Autodesk Inventor part; units mm, degrees
ref_plane "Work Plane1" through (0, 0, -15) normal (0, 0, 1) x (1, 0, 0)
ref_plane "YZ Plane" through (0, 0, 0) normal (1, 0, 0) x (0, 1, 0)
ref_plane "XZ Plane" through (0, 0, 0) normal (0, 1, 0) x (-1, 0, 0)
sketch "Sketch1" plane through (0, 0, 0) normal (0, 0, 1) x (1, 0, 0)
  line L0 (0, 0) -> (25, 0)
  line L1 (25, 0) -> (25, 40)
  line L2 (25, 40) -> (0, 40)
  line L3 (0, 40) -> (0, 0)
  dimension "d1" = 25
  dimension "d2" = 40
  dimension "d3" = 25
extrude "Extrusion1" add sketch "Sketch1" against normal blind 30
sketch "Sketch2" plane through (25, 0, 0) normal (1, 0, 0) x (0, 0, -1)
  line L0 (0, 0) -> (30, 0)
  circle A0 centre (15, 6.56) radius 2.46
extrude "Extrusion2" cut sketch "Sketch2" against normal blind 30
sketch "Sketch3" plane through (0, 0, 0) normal (-1, 0, 0) x (0, 0, 1)
  line L0 (0, 0) -> (-30, 0)
  line L1 (-25.05, 0) -> (-4.95, 0)
  line L2 (-4.95, 0) -> (-4.95, 33.12)
  line L3 (-4.95, 33.12) -> (-25.05, 33.12)
  line L4 (-25.05, 33.12) -> (-25.05, 0)
  dimension "d11" = 20.1
extrude "Extrusion3" cut sketch "Sketch3" against normal blind 20
sketch "Sketch4" plane through (0, 0, 0) normal (0, -1, 0) x (1, 0, 0)
  line L0 (20, -4.95) -> (20, -25.05)
  line L1 (20, -15) -> (25, -15)
  line L2 (25, 0) -> (25, -30)
  line L3 (20, -8.025) -> (25, -8.025)
  line L4 (25, -8.025) -> (25, -21.975)
  line L5 (25, -21.975) -> (20, -21.975)
  line L6 (20, -21.975) -> (20, -8.025)
  line L7 (20, -8.025) -> (25, -21.975) construction
  line L8 (25, -8.025) -> (20, -21.975) construction
  line L9 (25, -12.54) -> (25, -17.46)
  point P0 (0, 0)
  point P1 (22.5, -15)
  dimension "d14" = 13.95
extrude "Extrusion4" add sketch "Sketch4" along normal blind 15
sketch "Sketch5" plane through (20, 0, 0) normal (-1, 0, 0) x (0, 0, 1)
  circle A0 centre (-15, 6.56) radius 2.46
  circle A1 centre (-15, 6.56) radius 4.7025
  circle A2 centre (-15, 6.56) radius 2.46
  circle A3 centre (-15, 6.56) radius 2.46
  point P0 (0, 0)
  dimension "d17" = 9.405
extrude "Extrusion5" cut sketch "Sketch5" against normal blind 2.1
sketch "Sketch6" plane through (25, 0, 0) normal (1, 0, 0) x (0, 0, -1)
  circle A0 centre (15, 6.56) radius 4.7025
  line L0 (15, 6.56) -> (15, 23.56)
  circle A1 centre (15, 23.56) radius 2.46
  point P0 (0, 0)
  dimension "d20" = 17
  dimension "d21" = 4.92
extrude "Extrusion6" cut sketch "Sketch6" against normal blind 10 contours A1
sketch "Sketch7" plane through (20, 0, 0) normal (-1, 0, 0) x (0, 0, 1)
  circle A0 centre (-15, 23.56) radius 2.46
  circle A1 centre (-15, 23.56) radius 4.7025
  point P0 (0, 0)
  dimension "d24" = 9.405
extrude "Extrusion7" cut sketch "Sketch7" against normal blind 2.1
sketch "Sketch9" plane through (25, 0, 0) normal (1, 0, 0) x (0, 0, -1)
  circle A0 centre (15, 6.56) radius 2.46
  circle A1 centre (15, 6.56) radius 2.46
  circle A2 centre (15, 23.56) radius 2.46
  circle A3 centre (15, 23.56) radius 2.46
  line L0 (30, 40) -> (30, 0)
  line L1 (30, 0) -> (30, 40)
  line L2 (30, 40) -> (0, 40)
  line L3 (0, 40) -> (0, 0)
  line L4 (0, 0) -> (8.025, 0)
  line L5 (21.975, 0) -> (21.975, -15)
  line L6 (21.975, -15) -> (8.025, -15)
  line L7 (8.025, -15) -> (8.025, 0)
  line L8 (0, 0) -> (8.025, 0)
  line L9 (21.975, 0) -> (30, 0)
extrude "Extrusion8" add sketch "Sketch9" along normal blind 5
sketch "Sketch10" plane through (0, 40, 0) normal (0, 1, 0) x (1, 0, 0)
  line L0 (0, 30) -> (30, 30)
  line L1 (30, 0) -> (0, 0)
  line L2 (0, 30) -> (30, 30)
  line L3 (30, 30) -> (30, 0)
  line L4 (30, 0) -> (0, 0)
  line L5 (0, 0) -> (0, 30)
extrude "Extrusion9" add sketch "Sketch10" along normal blind 30
sketch "Sketch12" plane through (30, 0, 0) normal (1, 0, 0) x (0, 0, -1)
  circle A0 centre (15, 6.56) radius 2.46
  line L0 (15, 6.56) -> (15, 15.06)
  circle A1 centre (15, 15.06) radius 2.525
  point P0 (0, 0)
  dimension "d31" = 8.5
  dimension "d33" = 5.05
extrude "Extrusion10" cut sketch "Sketch12" against normal blind 30 contours A1
sketch "Sketch15" plane through (0, 0, -25.05) normal (-1, 0, 0) x (0, 0, 1)
  line L0 (0, 33.12) -> (20.1, 33.12)
  line L1 (20.1, 33.12) -> (20.1, 0)
  line L2 (0, 33.12) -> (20.1, 33.12)
  line L3 (20.1, 33.12) -> (20.1, 31.1)
  line L4 (20.1, 31.1) -> (0, 31.1)
  line L5 (0, 31.1) -> (0, 33.12)
  point P0 (25.05, 0)
  dimension "d57" = 2.02
extrude "Extrusion13" add sketch "Sketch15" against normal blind 20
sketch "Sketch17" plane through (0, 0, 0) normal (0, 0, 1) x (1, 0, 0)
  line L0 (0, 70) -> (30, 70)
  line L1 (30, 70) -> (50.0622, 90.0622)
  line L2 (30, 70) -> (80, 70) construction
  line L3 (11.9522, 97.2454) -> (0, 85.2932)
  line L4 (0, 70) -> (0, 85.2932)
  line L5 (0, 70) -> (0, 0)
  line L6 (0, 70) -> (30, 70)
  line L7 (10.923, 112.2849) -> (0, 120.567)
  line L8 (50.0622, 105.3553) -> (50.0622, 120.567)
  line L9 (50.0622, 105.3553) -> (50.0622, 90.0622)
  arc A0 (11.9522, 97.2454) -> (10.923, 112.2849) centre (4.8811, 104.3165) ccw
  line L10 (0, 150.567) -> (30, 150.567)
  line L11 (30, 150.567) -> (50.0622, 120.567)
  line L12 (5, 147.567) -> (0, 150.567)
  line L13 (5, 123.567) -> (0, 120.567)
  line L14 (5, 123.567) -> (10, 135.567)
  line L15 (10, 135.567) -> (5, 147.567)
  dimension "d61" = 45
  dimension "d62" = 32.0271
  dimension "d72" = 10
extrude "Extrusion14" add sketch "Sketch17" against normal blind 30
sketch "Sketch22" plane through (0, 0, 0) normal (0, 0, 1) x (1, 0, 0)
  line L0 (30, 0) -> (30, 70)
  line L1 (50.0622, 120.567) -> (50.0622, 90.0622)
  line L2 (30, 70) -> (50.0622, 90.0622)
  line L3 (50.0622, 90.0622) -> (50.0622, 120.567)
  line L4 (50.0622, 120.567) -> (30, 150.567)
  line L5 (50.0622, 120.567) -> (30, 150.567)
  line L6 (30, 150.567) -> (0, 150.567)
  line L7 (30, 150.567) -> (0, 150.567)
  line L8 (0, 150.567) -> (5, 147.567)
  line L9 (0, 150.567) -> (5, 147.567)
  line L10 (5, 147.567) -> (10, 135.567)
  line L11 (5, 147.567) -> (10, 135.567)
  line L12 (5, 123.567) -> (10, 135.567)
  line L13 (10, 135.567) -> (5, 123.567)
  line L14 (5, 123.567) -> (0, 120.567)
  line L15 (5, 123.567) -> (0, 120.567)
  line L16 (10.923, 112.2849) -> (0, 120.567)
  line L17 (0, 120.567) -> (10.923, 112.2849)
  line L18 (0, 85.2932) -> (11.9522, 97.2454)
  line L19 (11.9522, 97.2454) -> (0, 85.2932)
  line L20 (0, 85.2932) -> (0, 55.2932)
  line L21 (0, 0) -> (0, 85.2932)
  line L22 (0, 55.2932) -> (30, 55.2932)
  line L23 (30, 55.2932) -> (30, 70)
  arc A0 (11.9522, 97.2454) -> (10.923, 112.2849) centre (4.8811, 104.3165) ccw
  arc A1 (11.9522, 97.2454) -> (10.923, 112.2849) centre (4.8811, 104.3165) ccw
  dimension "d87" = 30
extrude "Extrusion15" add sketch "Sketch22" along normal blind 30
ref_plane "Work Plane1" through (0, 0, -15) normal (0, 0, 1) x (1, 0, 0)
mirror "Mirror1" about plane through (0, 0, -15) normal (0, 0, 1) of "Extrusion15"
properties part number "rec_c_24mm_x_90mm"
Source: CAD feature listing. Evaluate the final solid. Frame: model axes, mm. A direction names the side the tool comes from. Give positions to 0.01 mm unless a question says otherwise; leave off trailing zeros. Loops run counter-clockwise (first coordinate to the right, second up) from the corner with the lowest first, then second, coordinate; pieces in that order, holes last. Notation, with made-up numbers: (29, 20) -> (88, 20) arc R22 cw to (88, 36) -> close; hole circle Ø9 at (45.5, 24). An arc over 180 degrees is marked (long way). Put each result on its own line as item: value. Start each with the question number.
1) Contact query for flat-ended pins moving along their axis: P1, Ø6, axis at y = 4, z = -13.5, coming from the -X side; P2, Ø12, axis at y = 132.5, z = -12, coming from the +X side; P3, Ø24, axis at x = 15, z = 8.5, coming from the -Y side. Output: stop coordinate, or through.
2) Material intervals for probe 1 along Y at (x, z) = (28.25, -15) (3 decimals); probe 2 along Y at (x, z) = (21, -15) (1 decimal); probe 3 along Z at (x, y) = (26.5, 15.06) (3 decimals), sorted ascending.
3) Cut plane A-A (y = 15.06). Return loops of the section in (x, z) (3 decimals), then the cut area to 4 significant figures.
4) Cut plane C-C (z = 22.5). Return loops of the section in (x, y).
5) Draft query along Y for faces 1 (the face through (6.06, 91.353, -14.37)), 2 (the face through (15, 55.293, -45)), 3 (the face through (25.995, 7.502, -17.272)), 4 (the face through (30, 47, -14)). Return one class per face: released by +Y, released by -Y, zero draft, split by the parting line, or undercut.
6) Cut plane B-B (z = -15). State how many separate pieces and enclosed holes the cut face has, then the cut area to 3 significant figures.
7) Cut plane D-D (x = 32). Return loops of the section in (y, z), then the cut area to 3 significant figures.
8) Reachability of faces 5 (the face through (2.465, 122.046, -14.37)), 6 (the face through (21.035, 7.973, -10.515)), 7 (the face through (10, 16, -25.05)) from +Z, -Z, +X, -X, +Y, -Y: full face, straight path, thin tool, end or side. Return the list, or none.
Results are:
1. P1: stops at x = 20
1. P2: stops at x = 46.09
1. P3: stops at y = 0
2. probe 1: y = -15 to 4.1, 9.02 to 12.535, 17.585 to 21.1, 26.02 to 150.567
2. probe 2: y = -15 to 1.9, 11.3 to 12.5, 17.6 to 18.9, 28.3 to 150.6
2. probe 3: z = -30 to -17.525, -12.475 to 0
3. outline: (0, -30) -> (30, -30) -> (30, -17.525) -> (20, -17.525) -> (20, -25.05) -> (0, -25.05) -> close; (0, -4.95) -> (20, -4.95) -> (20, -12.475) -> (30, -12.475) -> (30, 0) -> (0, 0) -> close
3. area: 447.5 mm2
4. outline: (0, 55.29) -> (30, 55.29) -> (30, 70) -> (50.06, 90.06) -> (50.06, 120.57) -> (30, 150.57) -> (0, 150.57) -> (5, 147.57) -> (10, 135.57) -> (5, 123.57) -> (0, 120.57) -> (10.92, 112.28) arc R10 cw to (11.95, 97.25) -> (0, 85.29) -> close
5. face 1: undercut
5. face 2: released by -Y
5. face 3: undercut
5. face 4: zero draft
6. separate pieces: 4
6. enclosed holes: 0
6. area: 4,470 mm2
7. outline: (72, -60) -> (147.58, -60) -> (147.58, 30) -> (72, 30) -> close
7. area: 6,800 mm2
8. face 5: +Z, -Z, -X
8. face 6: -X
8. face 7: -X, -Y
